```python
from build123d import *

# Parameters (mm, degrees)
PAD_DEPTH = 3.5


with BuildPart() as part:
    # Sketch → Pad (new body)
    with BuildSketch(Plane.XY):
        with BuildLine():
            Line((-4.15, -0.25), (-4.15, 0.25))
            Line((-4.15, 0.25), (-4.1, 0.25))
            ThreePointArc((4.1, 0.25), (0, 4.35), (-4.1, 0.25))
            Line((4.1, 0.25), (4.15, 0.25))
            Line((4.15, 0.25), (4.15, -0.25))
            Line((4.15, -0.25), (4.1, -0.25))
            ThreePointArc((-4.1, -0.25), (0, -4.35), (4.1, -0.25))
            Line((-4.1, -0.25), (-4.15, -0.25))
        make_face()
    extrude(amount=PAD_DEPTH)

    # Sketch001 → Revolution (revolve)
    with BuildSketch(Plane.XZ):
        with BuildLine():
            Line((0, 0), (-4.3, 0))
            ThreePointArc((-4.3, 0), (-5.007107, -0.292893), (-5.3, -1))
            Line((-5.3, -1), (0, -1))
            Line((0, -1), (0, 0))
        make_face()
    revolve(axis=Axis((0, 0, 0), (0, 0, 1)))


solid = part.part
```
Work out the finished part from the listing and answer in its coordinate system (mm). A direction names the side the tool comes from. Round coordinates to 2 decimals unless told otherwise and drop trailing zeros. Write each loop counter-clockwise with the first axis right and the second up, starting at its lowest first coordinate (ties: lowest second). Pieces come first, ordered by that corner, then holes. Notation, with made-up numbers: (45.25, 85.5) -> (92.25, 85.5) arc R25 ccw to (92.25, 117.5) -> close; hole circle Ø10 at (82, 30.5). An arc over 180 degrees is marked (long way). Write each question's results on one line, items separated by ' | '.
Q1. Which of the six approach directions +Z, -Z, +X, -X, +Y, -Y give full straight-line access (tool end or side, diameter ignored) to faces 1 (the cylindrical face through (0.09, 4.35, 1.73)), 2 (the cylindrical face through (-0.09, -4.35, 1.73)), 3 (the flat face through (0, 0, -1))?
Data:
face 1: +Z, +Y | face 2: +Z, -Y | face 3: -Z, +X, -X, +Y, -Y
Q2. Straight lines are drawn through the part: line 1 along Z through (x, y) = (3.75, 2.25); line 2 along Y through (x, z) = (0, 2.4); line 3 along X through (y, z) = (2, 2.1). For each, find the intervals that lie inside material, in ascending order. Write a range as [from, to].
Data:
line 1: [-1, 0] | line 2: [-4.35, 4.35] | line 3: [-3.71, 3.71]
Q3. Flat-ended cylindrical pins translate along their axes: P1, Ø1, axis at y = -1.5, z = 3, coming from the -X side; P2, Ø1.5, axis at x = -4, z = 1, coming from the +Y side; P3, Ø1.5, axis at x = -0.5, z = 1.5, coming from the +Y side. Find the tip coordinate at first contact, or state that the pin passes through.
Data:
P1: x = -4.03 | P2: y = 2.75 | P3: y = 4.35
Q4. Section C-C, the plane z = -0.4 is taken. Write down the section's boundary in (x, y).
Data:
outline: circle Ø10.2 at (0, 0)
Q5. Section B-B, the plane x = 0 is taken. Write down the section's boundary in (y, z), then the cut area to 3 significant figures.
Data:
outline: (-5.3, -1) -> (5.3, -1) arc R1 ccw to (4.3, 0) -> (4.35, 0) -> (4.35, 3.5) -> (-4.35, 3.5) -> (-4.35, 0) -> (-4.3, 0) arc R1 ccw to start | area: 40.6 mm^2
Q6. Section A-A, the plane z = 2.8 is taken. Write down the section's boundary in (x, y), then the cut area to 3 significant figures.
Data:
outline: (-4.15, -0.25) -> (-4.1, -0.25) arc R4.1 ccw to (4.1, -0.25) -> (4.15, -0.25) -> (4.15, 0.25) -> (4.1, 0.25) arc R4.1 ccw to (-4.1, 0.25) -> (-4.15, 0.25) -> close | area: 57.0 mm^2
